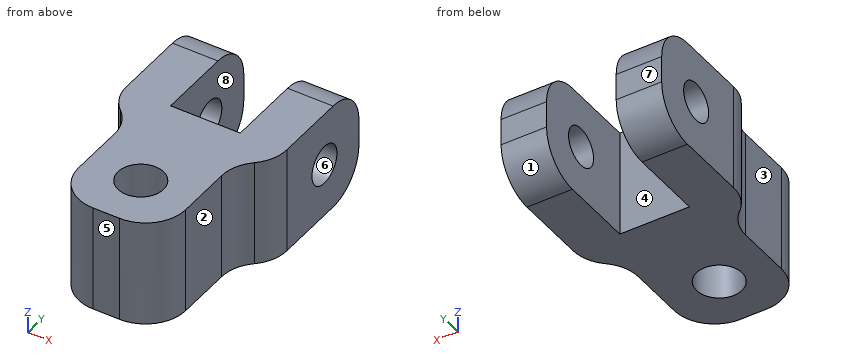
```python
from build123d import *

# Parameters (mm, degrees)
SKETCH_1_W          = 8
SKETCH_1_H          = 8
EXTRUDE_1_DEPTH     = 20
SKETCH_2_R          = 1.7
CUT_EXTRUDE_1_DEPTH = 23.978250586
SKETCH_4_W          = 2
SKETCH_4_H          = 8
EXTRUDE_3_DEPTH     = 10
SKETCH_5_W          = 5.2
SKETCH_5_H          = 8.5
CUT_EXTRUDE_2_DEPTH = 24.748684174
FILLET_1_R          = 3
SKETCH_6_R          = 1.45
CUT_EXTRUDE_3_DEPTH = 25.657656012
FILLET_2_R          = 3


with BuildPart() as part:
    # 草图1 → 凸台-拉伸1 (new body)
    with BuildSketch(Plane(origin=(0, 0, 0), x_dir=(1, 0, 0), z_dir=(0, 1, 0))):
        with Locations((4, -4)):
            Rectangle(SKETCH_1_W, SKETCH_1_H)
    extrude(amount=EXTRUDE_1_DEPTH)

    # 草图2 → 切除-拉伸1 (cut, through all)
    with BuildSketch(Plane.XY.offset(8)):
        with Locations((4, 4)):
            Circle(SKETCH_2_R)
    extrude(amount=-CUT_EXTRUDE_1_DEPTH, mode=Mode.SUBTRACT)

    # 草图4 → 凸台-拉伸3 (add)
    with BuildSketch(Plane(origin=(0, 20, 0), x_dir=(1, 0, 0), z_dir=(0, 1, 0))):
        with Locations((-1, -4)):
            Rectangle(SKETCH_4_W, SKETCH_4_H)
        with Locations((9, -4)):
            Rectangle(SKETCH_4_W, SKETCH_4_H)
    extrude(amount=-EXTRUDE_3_DEPTH)

    # 草图5 → 切除-拉伸2 (cut, through all)
    with BuildSketch(Plane.XY.offset(8)):
        with Locations((4, 15.75)):
            Rectangle(SKETCH_5_W, SKETCH_5_H)
    extrude(amount=-CUT_EXTRUDE_2_DEPTH, mode=Mode.SUBTRACT)

    # 圆角1
    # the kernel refuses this fillet: 3 mm, written as the material it adds along each edge
    with BuildSketch(Plane(origin=(8, 10, 8), x_dir=(0, -1, 0), z_dir=(0, 0, -1))) as fillet_1_piece_1:
        with BuildLine():
            CenterArc((2.828427125, -3), FILLET_1_R, 90, 70.528779366)
            Line((0, -2), (-0.056568542, -1.98))
            ThreePointArc((-0.056568542, -1.98), (-0.06, -1), (-0.06, 0))
            Line((-0.06, 0), (0, 0.06))
            Line((0, 0.06), (2.828427125, 0.06))
            Line((2.828427125, 0.06), (2.828427125, 0))
        make_face()
    extrude(amount=8)
    with BuildSketch(Plane(origin=(0, 10, 8), x_dir=(-1, 0, 0), z_dir=(0, 0, -1))) as fillet_1_piece_2:
        with BuildLine():
            CenterArc((3, -2.828427125), FILLET_1_R, 109.471220634, 70.528779366)
            Line((0, -2.828427125), (-0.06, -2.828427125))
            Line((-0.06, -2.828427125), (-0.06, 0))
            Line((-0.06, 0), (0, 0.06))
            ThreePointArc((0, 0.06), (1, 0.06), (1.98, 0.056568542))
            Line((1.98, 0.056568542), (2, 0))
        make_face()
    extrude(amount=8)

    # 草图6 → 切除-拉伸3 (cut, through all)
    with BuildSketch(Plane(origin=(10, 0, 0), x_dir=(0, 0, -1), z_dir=(1, 0, 0))):
        with Locations((-4, 16)):
            Circle(SKETCH_6_R)
    extrude(amount=-CUT_EXTRUDE_3_DEPTH, mode=Mode.SUBTRACT)

    # 圆角2
    fillet_2_edges = [part.edges().sort_by_distance(p)[0] for p in [
        (8.3, 20, 0),
        (-2, 10, 4),
        (10, 10, 4),
        (-0.3, 20, 0),
        (8.3, 20, 8),
        (8, 0, 4),
        (0, 0, 4),
        (-0.3, 20, 8),
    ]]
    fillet(fillet_2_edges, radius=FILLET_2_R)


solid = part.part
```
Here's how the part is built. I have some questions about the finished solid (model axes, mm). Face numbers are marked on the shaded views. A direction names the side the tool comes from. Round coordinates to 2 decimals unless told otherwise and drop trailing zeros. Order: outer loops, then holes, each group sorted by start corner. A loop starts at its lowest first (then second) coordinate and runs counter-clockwise, first axis right, second up. Notation, with made-up numbers: M 45.5,-39 L 104.5,-39 A27 ccw 104.5,-21 Z; hole C -23.5,80 d5. An arc over 180 degrees is marked long. Answer in a Markdown table with one row per item.
Item 1: If I drill on L1, parallel to Y at x = 4, z = 6.25; L2, parallel to X at y = 18.25, z = 5; L3, parallel to X at y = 6.5, z = 4.5, over which ranges is the centre line in solid material (lowest first)? Write a range as from..to.
A:
| item | result |
|---|---|
| L1 | y = 0..2.3, 5.7..11.5 |
| L2 | x = -2..1.4, 6.6..10 |
| L3 | x = 0..8 |
Item 2: For the marked faces 1, 2, 3 and 4, which set-ups out of +Z, -Z, +X, -X, +Y, -Y let a thin tool reach every point of the face, with its end or its side?
A:
| item | result |
|---|---|
| face 1 | -Z, +X, -X, +Y |
| face 2 | +Z, -Z, +X, -Y |
| face 3 | +Z, -Z, -X, -Y |
| face 4 | +Z, -Z, +Y |
Item 3: Imagine slicing it at B-B, the plane y = 4. Write out the boundary of the cut face in (x, z).
A:
| item | result |
|---|---|
| outline | M 0,0 L 2.3,0 L 2.3,8 L 0,8 Z; M 5.7,0 L 8,0 L 8,8 L 5.7,8 Z |
Item 4: I'm going to push flat-ended pins straight in: pin 1 (3.5 mm diameter, centred on y = 5.5, z = 4, fed in from +X); pin 2 (2 mm diameter, centred on x = 2, y = 15.5, fed in from +Z); pin 3 (1.7 mm diameter, centred on y = 16, z = 4, fed in from +X); pin 4 (4.5 mm diameter, centred on y = 5.5, z = 6, fed in from -X). Where does each tip first touch, or does it pass through?
A:
| item | result |
|---|---|
| pin 1 | stops at x = 8 |
| pin 2 | stops at z = 8 |
| pin 3 | passes through |
| pin 4 | stops at x = -0.06 |
Item 5: Imagine slicing it at A-A, the plane z = 4. Write out the boundary of the cut face in (x, y).
A:
| item | result |
|---|---|
| outline | M -2,11.64 A3 ccw -1,9.41 A3 cw 0,7.17 L 0,3 A3 ccw 3,0 L 5,0 A3 ccw 8,3 L 8,7.17 A3 cw 9,9.41 A3 ccw 10,11.64 L 10,14.55 L 6.6,14.55 L 6.6,11.5 L 1.4,11.5 L 1.4,14.55 L -2,14.55 Z; M -2,17.45 L 1.4,17.45 L 1.4,20 L -2,20 Z; M 6.6,17.45 L 10,17.45 L 10,20 L 6.6,20 Z; hole C 4,4 d3.4 |
Item 6: Imagine slicing it at C-C, the plane x = 4. Write out the boundary of the cut face in (y, z).
A:
| item | result |
|---|---|
| outline | M 0,0 L 2.3,0 L 2.3,8 L 0,8 Z; M 5.7,0 L 11.5,0 L 11.5,8 L 5.7,8 Z |
Item 7: Imagine slicing it at D-D, the plane y = 16. Write out the boundary of the cut face in (x, z).
A:
| item | result |
|---|---|
| outline | M -2,0 L 1.4,0 L 1.4,2.55 L -2,2.55 Z; M -2,5.45 L 1.4,5.45 L 1.4,8 L -2,8 Z; M 6.6,0 L 10,0 L 10,2.55 L 6.6,2.55 Z; M 6.6,5.45 L 10,5.45 L 10,8 L 6.6,8 Z |
Item 8: Thinking about a two-plate mould opening in Y: for the marked faces 5, 6, 7 and 8, which applies, +Y half, -Y half, draft (parallel to the pull), parting line (faces both ways), or undercut?
A:
| item | result |
|---|---|
| face 5 | -Y half |
| face 6 | undercut |
| face 7 | +Y half |
| face 8 | draft |
